Work out the finished part from the listing and answer in its coordinate system (mm). Face numbers are marked on the shaded views. A direction names the side the tool comes from. Give positions to 0.01 mm unless a question says otherwise; leave off trailing zeros. Write each loop counter-clockwise with the first axis right and the second up, starting at its lowest first coordinate (ties: lowest second). Pieces come first, ordered by that corner, then holes.
1) Determine the mould class of the marked faces 4, 5, 6 and 7 for opening direction X: pulls with the +X half, pulls with the -X half, needs draft (parallel to the pull), parting line crosses it, or undercut.
2) Find section C-C (x = -3.75). Determine the outline of the cut face in (y, z) (3 decimals).
3) Find section B-B (y = 0.25). Determine the outline of the cut face in (x, z) (3 decimals), plus the area to 3 significant figures.
4) A tool of negligible diameter and unlimited length cuts with its end or side. For the marked faces 1, 2 and 3, from which of +Z, -Z, +X, -X, +Y, -Y can it reach the whole face along a straight path? Write none if from no direction.
5) Straight lines are drawn through the part: probe 1 along X at (y, z) = (1.15, 0) (3 decimals); probe 2 along Z at (x, y) = (-2.25, 12.5); probe 3 along X at (y, z) = (1.25, -2.5). For each, find the intervals that lie inside material, in ascending order.
6) Given pin 1 Ø1.8 at (x, z) = (-3.5, 0) entering from +Y, flat-ended and moving along its own axis, determine where the tip first touches the part or whether it passes through.
7) Find section A-A (y = 8.25). Determine the outline of the cut face in (x, z) (3 decimals).
```python
from build123d import *

# Parameters (mm, degrees)
BOSS_EXTRUDE1_DEPTH      = 16
SHELL1_T                 = -0.5
SHELL1_THICKNESS_2_DEPTH = 6.5
SKETCH2_R                = 3
CUT_EXTRUDE1_DEPTH       = 1.5
SKETCH3_R                = 2.125
BOSS_EXTRUDE2_DEPTH      = 4.5
SKETCH4_R                = 2.125
BOSS_EXTRUDE3_DEPTH      = 8
FILLET1_R                = 1


with BuildPart() as part:
    # Sketch1 → Boss-Extrude1 (new body)
    with BuildSketch(Plane(origin=(0, 0, 0), x_dir=(1, 0, 0), z_dir=(0, 1, 0))):
        Polygon((7.75, 1.5), (5.25, 4), (-7.75, 4), (-7.75, -4), (5.25, -4), (7.75, -1.5), align=None)
    extrude(amount=BOSS_EXTRUDE1_DEPTH)

    # Shell1
    shell1_openings = [part.faces().sort_by_distance(p)[0] for p in [
        (-0.367126681, 16, 0),
    ]]
    offset(amount=SHELL1_T, openings=shell1_openings, kind=Kind.INTERSECTION)

    # Shell1 thickness 2 face (on inner face of the shell) → Shell1 thickness 2 (add)
    with BuildSketch(Plane(origin=(-0.328403857, 0.5, 0), x_dir=(0, 0, -1), z_dir=(0, -1, 0))):
        Polygon((-1.292893219, 7.578403857), (1.292893219, 7.578403857), (3.5, 5.371297076), (3.5, -6.921596143), (-3.5, -6.921596143), (-3.5, 5.371297076), align=None)
    extrude(amount=-SHELL1_THICKNESS_2_DEPTH)

    # Sketch2 → Cut-Extrude1 (cut)
    with BuildSketch(Plane.XZ):
        with Locations(Location((-3.75, 0, 0), (0, 0, 270))):
            Circle(SKETCH2_R)
        with Locations(Location((3.75, 0, 0), (0, 0, 90))):
            Circle(SKETCH2_R)
    extrude(amount=-CUT_EXTRUDE1_DEPTH, mode=Mode.SUBTRACT)

    # Sketch3 → Boss-Extrude2 (add)
    with BuildSketch(Plane.XZ.offset(-1.5)):
        with Locations(Location((-3.75, 0, 0), (0, 0, 270))):
            Circle(SKETCH3_R)
        with Locations(Location((3.75, 0, 0), (0, 0, 90))):
            Circle(SKETCH3_R)
    extrude(amount=BOSS_EXTRUDE2_DEPTH)

    # Sketch4 → Boss-Extrude3 (add)
    with BuildSketch(Plane(origin=(0, 7, 0), x_dir=(1, 0, 0), z_dir=(0, 1, 0))):
        with Locations(Location((-3.75, 0, 0), (0, 0, 90))):
            Circle(SKETCH4_R)
        with Locations(Location((3.75, 0, 0), (0, 0, 270))):
            Circle(SKETCH4_R)
    extrude(amount=BOSS_EXTRUDE3_DEPTH)

    # Fillet1
    fillet1_edges = [part.edges().sort_by_distance(p)[0] for p in [
        (-3.75, 15, 2.125),
        (3.75, 15, -2.125),
    ]]
    fillet(fillet1_edges, radius=FILLET1_R)


solid = part.part
```
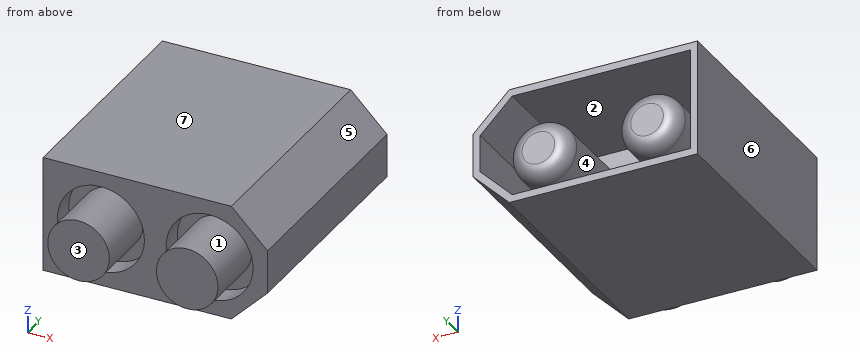
Results:
1. face 4: undercut
1. face 5: pulls with the +X half
1. face 6: pulls with the -X half
1. face 7: needs draft
2. outline: (-3, -2.125) - (1.5, -2.125) - (1.5, -3) - (0, -3) - (0, -4) - (16, -4) - (16, -3.5) - (7, -3.5) - (7, -2.125) - (14, -2.125) arc R1 ccw to (15, -1.125) - (15, 1.125) arc R1 ccw to (14, 2.125) - (7, 2.125) - (7, 3.5) - (16, 3.5) - (16, 4) - (0, 4) - (0, 3) - (1.5, 3) - (1.5, 2.125) - (-3, 2.125) - close
3. outline: (-7.75, -4) - (5.25, -4) - (7.75, -1.5) - (7.75, 1.5) - (5.25, 4) - (-7.75, 4) - close; circle Ø4.25 at (-3.75, 0); circle Ø4.25 at (3.75, 0); hole circle Ø6 at (-3.75, 0); hole circle Ø6 at (3.75, 0)
3. area: 89.6 mm2
4. face 1: -Y
4. face 2: +Y
4. face 3: +Z, -Z, +X, -X, -Y
5. probe 1: x = -7.75 to -6.75, -5.875 to -1.625, -0.75 to 0.75, 1.625 to 5.875, 6.75 to 7.75
5. probe 2: z = -4 to -3.5, -1.51 to 1.51, 3.5 to 4
5. probe 3: x = -7.75 to -5.41, -2.09 to 2.09, 5.41 to 6.75
6. pin 1: stops at y = 15
7. outline: (-7.75, -4) - (5.25, -4) - (7.75, -1.5) - (7.75, 1.5) - (5.25, 4) - (-7.75, 4) - close; circle Ø4.25 at (-3.75, 0); circle Ø4.25 at (3.75, 0); hole (-7.25, -3.5) - (5.043, -3.5) - (7.25, -1.293) - (7.25, 1.293) - (5.043, 3.5) - (-7.25, 3.5) - close
